The listing builds one solid part. Answer for the finished solid, in the listing's coordinates (mm). A direction names the side the tool comes from. Coordinates: 2 decimals unless noted, no trailing zeros. Loops run counter-clockwise (first coordinate to the right, second up) from the corner with the lowest first, then second, coordinate; pieces in that order, holes last. Notation, with made-up numbers: (83, 42.5) -> (138, 42.5) arc R19 ccw to (138, 71.5) -> close; hole circle Ø3 at (78.25, -20.75). An arc over 180 degrees is marked (long way). Answer in a Markdown table with one row per item.
```python
from build123d import *

# Parameters (mm, degrees)
F1_DEPTH = 63.5
F0_W     = 25.3298562567
F0_H     = 19.05
F2_DEPTH = 25.4
F3_DEPTH = 7.9375


with BuildPart() as f1:
    # F0 (on Front) → F1 (new body, symmetric)
    with BuildSketch(Plane.XZ):
        Polygon((-41.275, 9.525), (-41.275, -9.525), (41.275, -9.525), (41.275, 9.525), (22.225, 9.525), align=None)
    extrude(amount=F1_DEPTH, both=True)

    # F0 (on Front) → F2 (join, symmetric)
    with BuildSketch(Plane.XZ):
        with BuildLine():
            Line((22.225, 9.525), (41.275, 9.525))
            Line((41.275, 9.525), (41.275, 27.0002))
            ThreePointArc((41.275, 27.0002), (45.9246798487, 38.2255201513), (57.15, 42.8752))
            Line((57.15, 42.8752), (60.325, 42.8752))
            Line((60.325, 42.8752), (60.325, 61.9252))
            Line((60.325, 61.9252), (57.15, 61.9252))
            add(Edge.make_bspline(
                [(52.5566804935, 61.6218267803), (54.0650417221, 61.7326720686), (55.596048457, 61.833893026), (57.15, 61.9252)],
                knots=[109.2974079023, 109.2974079023, 109.2974079023, 109.2974079023, 111.5045361635, 111.5045361635, 111.5045361635, 111.5045361635], degree=3))
            ThreePointArc((52.5566804935, 61.6218267803), (30.8804614738, 50.0146947939), (22.225, 27.0002))
            Line((22.225, 27.0002), (22.225, 9.525))
        make_face()
        with Locations((72.9899281284, 52.4002)):
            Rectangle(F0_W, F0_H)
    extrude(amount=F2_DEPTH, both=True)

    # F0 (on Front) → F3 (join, symmetric)
    with BuildSketch(Plane.XZ):
        with BuildLine():
            add(Edge.make_bspline(
                [(-41.275, 9.525), (-41.2995623579, 27.0424108455), (-22.1376521166, 56.1327471898), (52.5566804935, 61.6218267803)],
                knots=[0, 0, 0, 0, 109.2974079023, 109.2974079023, 109.2974079023, 109.2974079023], degree=3))
            Line((-41.275, 9.525), (22.225, 9.525))
            Line((22.225, 9.525), (22.225, 27.0002))
            ThreePointArc((22.225, 27.0002), (30.8804614738, 50.0146947939), (52.5566804935, 61.6218267803))
        make_face()
    extrude(amount=F3_DEPTH, both=True)

    # F0 (on Front) → F4 (revolve)
    with BuildSketch(Plane.XZ):
        Polygon((85.6548562567, 66.675), (85.6548562567, 61.9252), (85.6548562567, 42.8752), (85.6548562567, 38.1), (111.125, 38.1), (111.125, 66.675), align=None)
    revolve(axis=Axis((85.6548562567, 0, 52.3875), (0, 0, 1)))


solid = f1.part
```
Item 1: A cutting plane is placed at B-B, the plane y = 33.5. Determine the outline of the cut face in (x, z) (3 decimals).
Findings below:
| item | result |
|---|---|
| outline | (-41.275, -9.525) -> (41.275, -9.525) -> (41.275, 9.525) -> (-41.275, 9.525) -> close |
Item 2: A cutting plane is placed at A-A, the plane z = 7.5. Determine the outline of the cut face in (x, y) (3 decimals).
Findings below:
| item | result |
|---|---|
| outline | (-41.275, -63.5) -> (41.275, -63.5) -> (41.275, 63.5) -> (-41.275, 63.5) -> close |
Item 3: A tool of negligible diameter and unlimited length cuts with its end or side. For faces 1 (the face through (-4, -7.938, 30)), 2 (the face through (86, 0, 38.1)), from which of +Z, -Z, +X, -X, +Y, -Y can it reach the whole face along a straight path? Write none if from no direction.
Findings below:
| item | result |
|---|---|
| face 1 | +Z, -X, -Y |
| face 2 | -Z, +X, +Y, -Y |
Item 4: Find the intervals of material crossed by probe 1 along X at (y, z) = (46, -3.5) (3 decimals); probe 2 along X at (y, z) = (7, 11) (1 decimal); probe 3 along Z at (x, y) = (-29, 8.5) (3 decimals), in increasing order.
Findings below:
| item | result |
|---|---|
| probe 1 | x = -41.275 to 41.275 |
| probe 2 | x = -41.2 to 41.3 |
| probe 3 | z = -9.525 to 9.525 |
Item 5: Flat-ended cylindrical pins translate along their axes: pin 1 Ø1.5 at (y, z) = (3, 40.5) entering from -X; pin 2 Ø5 at (x, z) = (-2, 53) entering from -Y; pin 3 Ø14 at (y, z) = (12.5, 20) entering from -X. Find the tip coordinate at first contact, or state that the pin passes through.
Findings below:
| item | result |
|---|---|
| pin 1 | stops at x = -22.84 |
| pin 2 | stops at y = -7.94 |
| pin 3 | stops at x = -40.75 |
